Design review of the part built by this model. Coordinates are the model's own, in mm. A direction names the side the tool comes from. Coordinates: 2 decimals unless noted, no trailing zeros. Order: outer loops, then holes, each group sorted by start corner. A loop starts at its lowest first (then second) coordinate and runs counter-clockwise, first axis right, second up. Notation, with made-up numbers: M 69,24.25 L 80,24.25 A12 cw 80,31.25 Z; hole C 26,28 d2. An arc over 180 degrees is marked long. Answer in a Markdown table with one row per item.
from build123d import *

# Parameters (mm, degrees)
SKETCH1_W           = 78
SKETCH1_H           = 50
SKETCH1_W_2         = 68
SKETCH1_H_2         = 38
BOSS_EXTRUDE1_DEPTH = 40
FILLET1_R           = 3
SKETCH2_R           = 3
CUT_EXTRUDE1_DEPTH  = 40
SKETCH3_R           = 2.5
CUT_EXTRUDE2_DEPTH  = 40
SKETCH4_R           = 1.475
CUT_EXTRUDE3_DEPTH  = 50


with BuildPart() as part:
    # Sketch1 → Boss-Extrude1 (new body)
    with BuildSketch(Plane(origin=(0, 0, 0), x_dir=(1, 0, 0), z_dir=(0, 1, 0))):
        with Locations((24.581369455, 5.203792641)):
            Rectangle(SKETCH1_W, SKETCH1_H)
        with Locations((24.581369455, 5.203792641)):
            Rectangle(SKETCH1_W_2, SKETCH1_H_2, mode=Mode.SUBTRACT)
    extrude(amount=BOSS_EXTRUDE1_DEPTH)

    # Fillet1
    fillet1_edges = [part.edges().sort_by_distance(p)[0] for p in [
        (58.581369455, 20, -24.203792641),
        (-9.418630545, 20, -24.203792641),
        (-9.418630545, 20, 13.796207359),
        (58.581369455, 20, 13.796207359),
        (-14.418630545, 20, 19.796207359),
        (-14.418630545, 20, -30.203792641),
        (63.581369455, 20, -30.203792641),
        (63.581369455, 20, 19.796207359),
    ]]
    fillet(fillet1_edges, radius=FILLET1_R)

    # Sketch2 → Cut-Extrude1 (cut)
    with BuildSketch(Plane(origin=(63.581369455, 0, 0), x_dir=(0, 0, -1), z_dir=(1, 0, 0))):
        with Locations((5.203792641, 20)):
            Circle(SKETCH2_R)
    extrude(amount=-CUT_EXTRUDE1_DEPTH, mode=Mode.SUBTRACT)

    # Sketch3 → Cut-Extrude2 (cut)
    with BuildSketch(Plane.ZY.offset(14.418630545)):
        with Locations((-5.203792641, 20)):
            Circle(SKETCH3_R)
    extrude(amount=-CUT_EXTRUDE2_DEPTH, mode=Mode.SUBTRACT)

    # Sketch4 → Cut-Extrude3 (cut)
    with BuildSketch(Plane(origin=(0, 0, -30.203792641), x_dir=(-1, 0, 0), z_dir=(0, 0, -1))):
        with Locations((-24.581369455, 30)):
            Circle(SKETCH4_R)
    extrude(amount=-CUT_EXTRUDE3_DEPTH, mode=Mode.SUBTRACT)


solid = part.part
(1) For faces 1 (the flat face through (24, 40, 17)), 2 (the cylindrical face through (61.116, 17.071, -4.553)), 3 (the flat face through (58.581, 20, -9)), list the 3-axis set-ups (+Z, -Z, +X, -X, +Y, -Y) from which the entire face can be reached by the end or side of a thin tool; tool diameter is ignored.
Return value:
| item | result |
|---|---|
| face 1 | +Z, -Z, +X, -X, +Y |
| face 2 | +X |
| face 3 | +Y, -Y |
(2) Add section A-A, the plane y = 20. Give the boundary of the cut face in (x, z).
Return value:
| item | result |
|---|---|
| outline | M -14.42,-27.2 A3 ccw -11.42,-30.2 L 60.58,-30.2 A3 ccw 63.58,-27.2 L 63.58,-8.2 L 58.58,-8.2 L 58.58,-21.2 A3 cw 55.58,-24.2 L -6.42,-24.2 A3 cw -9.42,-21.2 L -9.42,-7.7 L -14.42,-7.7 Z; M -14.42,-2.7 L -9.42,-2.7 L -9.42,10.8 A3 cw -6.42,13.8 L 55.58,13.8 A3 cw 58.58,10.8 L 58.58,-2.2 L 63.58,-2.2 L 63.58,16.8 A3 ccw 60.58,19.8 L -11.42,19.8 A3 ccw -14.42,16.8 Z |
(3) Add section D-D, the plane y = 10. Give the boundary of the cut face in (x, z), and give its area (3 significant figures).
Return value:
| item | result |
|---|---|
| outline | M -14.42,-27.2 A3 ccw -11.42,-30.2 L 60.58,-30.2 A3 ccw 63.58,-27.2 L 63.58,16.8 A3 ccw 60.58,19.8 L -11.42,19.8 A3 ccw -14.42,16.8 Z; hole M -9.42,-21.2 A3 ccw -6.42,-24.2 L 55.58,-24.2 A3 ccw 58.58,-21.2 L 58.58,10.8 A3 ccw 55.58,13.8 L -6.42,13.8 A3 ccw -9.42,10.8 Z |
| area | 1,320 mm2 |
(4) For line 1 along Z through (x, y) = (14, 21); line 2 along X through (y, z) = (5, -15.5); line 3 along X through (y, z) = (17.5, -23.5), list the stretches that pass through material, from the lowest coordinate up. Write a range as from..to.
Return value:
| item | result |
|---|---|
| line 1 | z = -30.2..-24.2, 13.8..19.8 |
| line 2 | x = -14.42..-9.42, 58.58..63.58 |
| line 3 | x = -14.42..-8.35, 57.51..63.58 |
(5) Draft analysis for pull direction Z (two halves, no side actions). For faces 4 (the flat face through (-14.419, 24, -5)), 5 (the cylindrical face through (57.68, 20.28, 12.94)), 6 (the flat face through (24, 20, 19.796)), state which applies: pulls with the +Z half, pulls with the -Z half, needs draft (parallel to the pull), parting line crosses it, or undercut.
Return value:
| item | result |
|---|---|
| face 4 | needs draft |
| face 5 | undercut |
| face 6 | pulls with the +Z half |
(6) Add section B-B, the plane z = -18. Give the boundary of the cut face in (x, y), and give its area (3 significant figures).
Return value:
| item | result |
|---|---|
| outline | M -14.42,0 L -9.42,0 L -9.42,40 L -14.42,40 Z; M 58.58,0 L 63.58,0 L 63.58,40 L 58.58,40 Z |
| area | 400 mm2 |
(7) Add section C-C, the plane x = 11. Give the boundary of the cut face in (y, z).
Return value:
| item | result |
|---|---|
| outline | M 0,-30.2 L 40,-30.2 L 40,-24.2 L 0,-24.2 Z; M 0,13.8 L 40,13.8 L 40,19.8 L 0,19.8 Z |
